For this review, use the dimensioned drawing (mm, ordinates from the lowest corner) and the shaded views. A direction names the side the tool comes from. Coordinates: 2 decimals unless noted, no trailing zeros. Write each loop counter-clockwise with the first axis right and the second up, starting at its lowest first coordinate (ties: lowest second). Pieces come first, ordered by that corner, then holes.
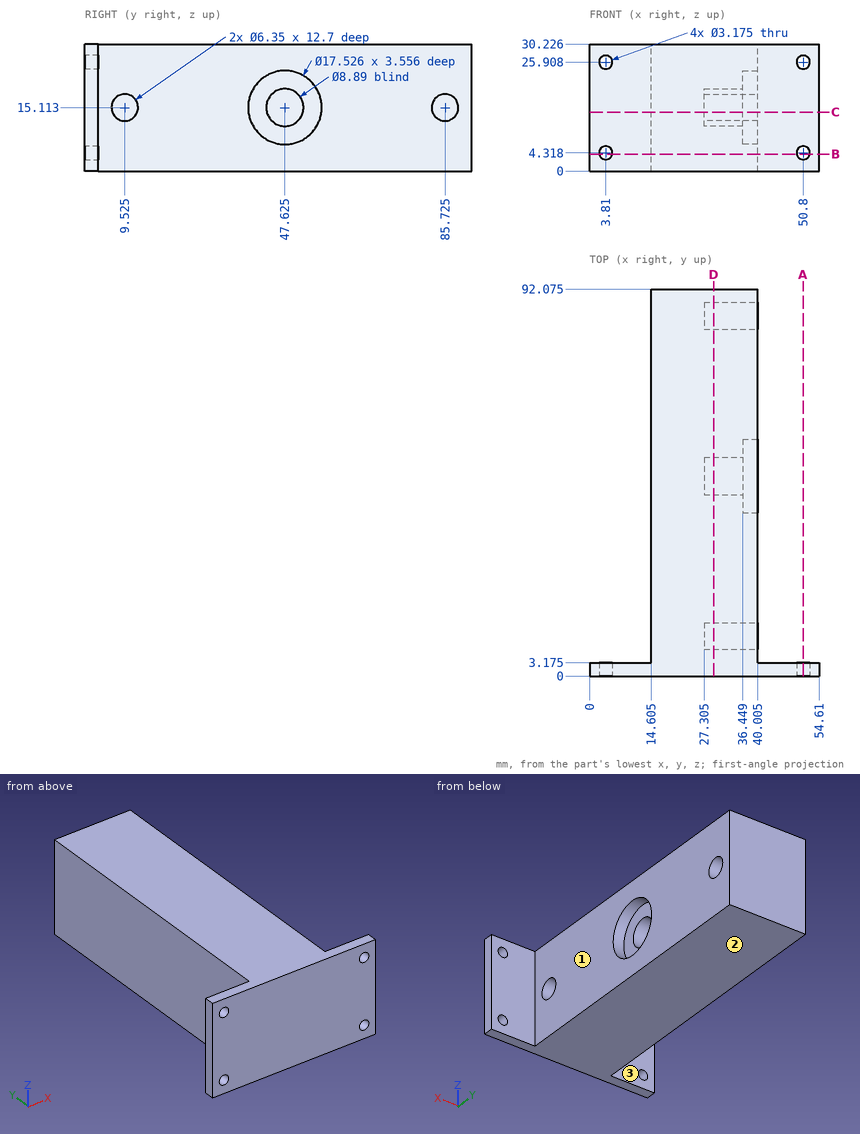
(1) Insertion check: pin 1 Ø7.5 at (y, z) = (85.725, 15.113) entering from +X (3 decimals); pin 2 Ø10.5 at (y, z) = (47.625, 15.113) entering from -X (3 decimals); pin 3 Ø1.9 at (x, z) = (3.81, 4.318) entering from +Y; pin 4 Ø1 at (x, z) = (11, 15.5) entering from +Y (3 decimals). Each pin has a flat end and moves straight along its axis. Give the tip position at first contact, or say it passes through.
(2) Consider section A-A (x = 50.8). Give the boundary of the cut face in (y, z) (1 decimal), plus the area to 3 significant figures.
(3) Consider section D-D (x = 29.5). Give the boundary of the cut face in (y, z) (3 decimals).
(4) For the marked faces 1, 2 and 3, list the 3-axis set-ups (+Z, -Z, +X, -X, +Y, -Y) from which the entire face can be reached by the end or side of a thin tool; tool diameter is ignored.
(5) Wall thickness on line 1 (X direction, y = 4, z = 19.5) (3 decimals); line 2 (Y direction, x = 43, z = 19) (3 decimals); line 3 (X direction, y = 45, z = 19.5) (3 decimals): over which ranges is each line inside the solid? List them lowest first.
(6) Consider section C-C (z = 14). Give the boundary of the cut face in (x, y) (3 decimals), plus the area to 3 significant figures.
(7) Consider section B-B (z = 4). Give the boundary of the cut face in (x, y) (3 decimals).
Results:
1. pin 1: stops at x = 40.005
1. pin 2: stops at x = 14.605
1. pin 3: passes through
1. pin 4: stops at y = 3.175
2. outline: (0, 0) - (3.2, 0) - (3.2, 2.7) - (0, 2.7) - close; (0, 5.9) - (3.2, 5.9) - (3.2, 24.3) - (0, 24.3) - close; (0, 27.5) - (3.2, 27.5) - (3.2, 30.2) - (0, 30.2) - close
2. area: 75.8 mm2
3. outline: (0, 0) - (92.075, 0) - (92.075, 30.226) - (0, 30.226) - close; hole circle Ø6.35 at (9.525, 15.113); hole circle Ø8.89 at (47.625, 15.113); hole circle Ø6.35 at (85.725, 15.113)
4. face 1: +Z, -Z, +X, +Y
4. face 2: -Z, +X, -X, +Y, -Y
4. face 3: +Z, -Z, -X, +Y
5. line 1: x = 14.605 to 40.005
5. line 2: y = 0 to 3.175
5. line 3: x = 14.605 to 36.449
6. outline: (0, 0) - (54.61, 0) - (54.61, 3.175) - (40.005, 3.175) - (40.005, 6.551) - (27.305, 6.551) - (27.305, 12.499) - (40.005, 12.499) - (40.005, 38.933) - (36.449, 38.933) - (36.449, 43.322) - (27.305, 43.322) - (27.305, 51.928) - (36.449, 51.928) - (36.449, 56.317) - (40.005, 56.317) - (40.005, 82.751) - (27.305, 82.751) - (27.305, 88.699) - (40.005, 88.699) - (40.005, 92.075) - (14.605, 92.075) - (14.605, 3.175) - (0, 3.175) - close
6. area: 2,140 mm2
7. outline: (0, 0) - (2.255, 0) - (2.255, 3.175) - (0, 3.175) - close; (5.365, 0) - (49.245, 0) - (49.245, 3.175) - (40.005, 3.175) - (40.005, 92.075) - (14.605, 92.075) - (14.605, 3.175) - (5.365, 3.175) - close; (52.355, 0) - (54.61, 0) - (54.61, 3.175) - (52.355, 3.175) - close
